```python
from build123d import *

# Parameters (mm, degrees)
F0_R     = 29.4761945826
F0_R_2   = 15.4337989403
F0_R_3   = 7.4174177389
F1_DEPTH = 7.62
F2_DEPTH = 10.16
F3_DEPTH = 25.4


with BuildPart() as f1:
    # F0 (on Front) → F1 (new body)
    with BuildSketch(Plane.XZ):
        Circle(F0_R)
        Circle(F0_R_2, mode=Mode.SUBTRACT)
        Circle(F0_R_2)
        Circle(F0_R_3, mode=Mode.SUBTRACT)
        Circle(F0_R_3)
    extrude(amount=F1_DEPTH)

    # F0 (on Front) → F2 (join)
    with BuildSketch(Plane.XZ):
        Circle(F0_R_2)
        Circle(F0_R_3, mode=Mode.SUBTRACT)
        Circle(F0_R_3)
    extrude(amount=-F2_DEPTH)

    # F0 (on Front) → F3 (join)
    with BuildSketch(Plane.XZ):
        Circle(F0_R_3)
    extrude(amount=-F3_DEPTH)


solid = f1.part
```
Could you check a few things on this model? Use its own coordinates, in mm. A direction names the side the tool comes from. Round coordinates to 2 decimals unless told otherwise and drop trailing zeros. Write each loop counter-clockwise with the first axis right and the second up, starting at its lowest first coordinate (ties: lowest second). Pieces come first, ordered by that corner, then holes.
(1) Suppose I cut it at A-A on x = 0. Write out the boundary of the cut face in (y, z).
Findings below:
outline: (-7.62, -29.48) - (0, -29.48) - (0, -15.43) - (10.16, -15.43) - (10.16, -7.42) - (25.4, -7.42) - (25.4, 7.42) - (10.16, 7.42) - (10.16, 15.43) - (0, 15.43) - (0, 29.48) - (-7.62, 29.48) - close
(2) If I drill on probe 1 along Y at (x, z) = (21.5, 3.5); probe 2 along Z at (x, y) = (6, 8); probe 3 along X at (y, z) = (7.5, -13.5), over which ranges is the centre line in solid material (lowest first)?
Findings below:
probe 1: y = -7.62 to 0
probe 2: z = -14.22 to 14.22
probe 3: x = -7.48 to 7.48
(3) For pin 1 (1 mm diameter, centred on x = -23.5, y = -4, fed in from -Z); pin 2 (8 mm diameter, centred on x = -14.5, z = 16.5, fed in from +Y); pin 3 (8 mm diameter, centred on y = 19, z = -1.5, fed in from +X), each with a flat end and sliding along its axis, tell me the tip position at first contact or that it passes through.
Findings below:
pin 1: stops at z = -18.43
pin 2: stops at y = 0
pin 3: stops at x = 7.42
(4) Suppose I cut it at D-D on z = -14. Write out the boundary of the cut face in (x, y).
Findings below:
outline: (-25.94, -7.62) - (25.94, -7.62) - (25.94, 0) - (6.5, 0) - (6.5, 10.16) - (-6.5, 10.16) - (-6.5, 0) - (-25.94, 0) - close
(5) Suppose I cut it at B-B on z = 0. Write out the boundary of the cut face in (x, y).
Findings below:
outline: (-29.48, -7.62) - (29.48, -7.62) - (29.48, 0) - (15.43, 0) - (15.43, 10.16) - (7.42, 10.16) - (7.42, 25.4) - (-7.42, 25.4) - (-7.42, 10.16) - (-15.43, 10.16) - (-15.43, 0) - (-29.48, 0) - close
(6) Which directions (+Z, -Z, +X, -X, +Y, -Y) give clear straight access to the entire face, cutting with the end or side of a thin tool? Please do faces 1 (the face through (14.72, 5.01, 4.64)), 2 (the face through (0, 25.4, 0)).
Findings below:
face 1: +Y
face 2: +Z, -Z, +X, -X, +Y
(7) Suppose I cut it at C-C on y = 2. Write out the boundary of the cut face in (x, z), and give its area (3 significant figures).
Findings below:
outline: circle Ø30.87 at (0, 0)
area: 748 mm2
